Drawing for the job (mm, zero at the part's lowest x, y, z). A direction names the side the tool comes from. Give positions to 0.01 mm unless a question says otherwise; leave off trailing zeros. Loops run counter-clockwise (first coordinate to the right, second up) from the corner with the lowest first, then second, coordinate; pieces in that order, holes last. Notation, with made-up numbers: (52, -3) - (74, -3) arc R14 ccw to (74, 1) - close; hole circle Ø8 at (13, -28.75). An arc over 180 degrees is marked (long way). Return JSON: item names as keys, results as strings. Group by question number.
1) 3-axis set-ups, long thin cutter, end or side, ignore diameter. For the marked faces 4 and 5: which of +Z, -Z, +X, -X, +Y, -Y reach the whole face in a straight line?
2) Slice it at A-A (z = 41.5). List the corners of the cut face in (x, y).
3) Slice it at C-C (y = 70). List the corners of the cut face in (x, z).
4) Slice it at B-B (x = 12.75). List the corners of the cut face in (y, z).
5) Drop flat-ended pins along their axis: pin 1 (8 mm diameter, centred on y = 73.5, z = 39.5, fed in from +X); pin 2 (5 mm diameter, centred on x = 3, z = 40.5, fed in from -Y). Give the stop position or say it passes through.
6) Mould opens along Y. For the marked faces 1, 2 and 3 say: released by +Y, released by -Y, zero draft, split by the parting line, or undercut.
7) Drill centre lines: probe 1 along Z at (x, y) = (11, 53.5); probe 2 along Y at (x, z) = (5, 90); probe 3 along X at (y, z) = (74, 47). Where is each one in solid material? Low to high. Write a range as from..to.
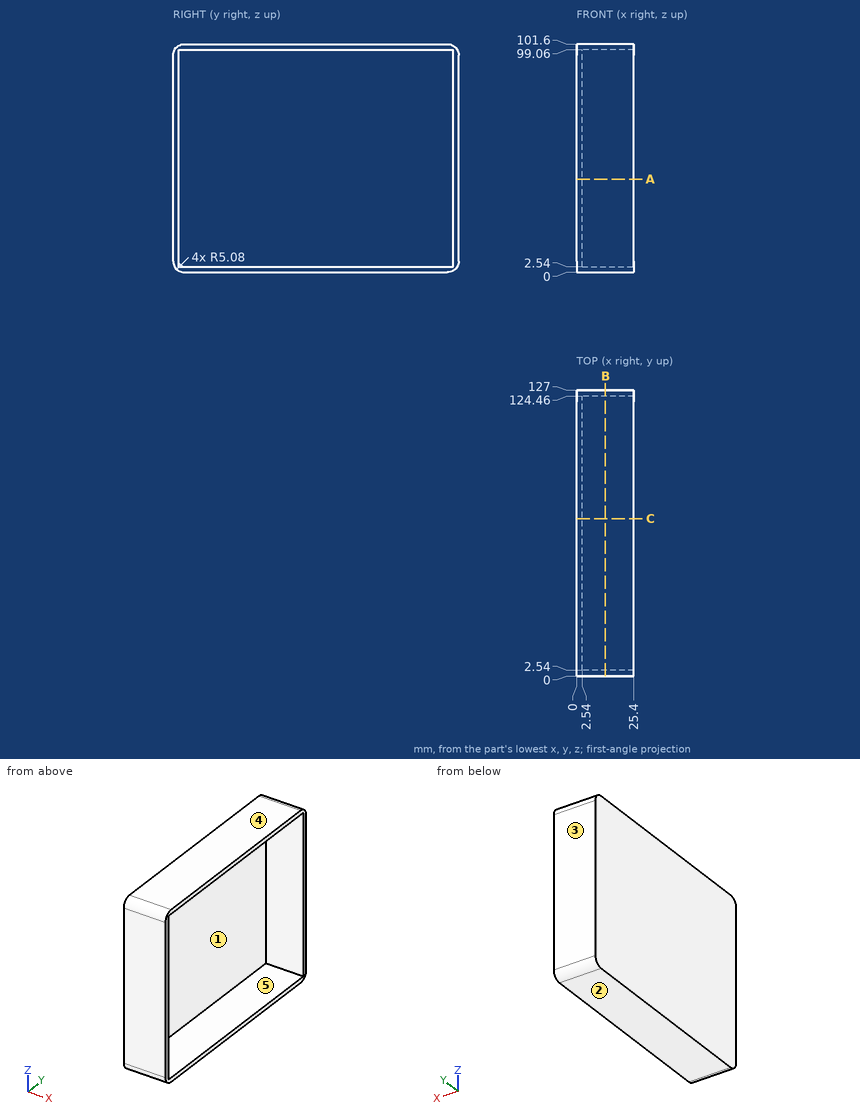
Results:
{
 "1": {"face 4": "+Z, +X, -X, +Y, -Y", "face 5": "+X"},
 "2": {"outline": "(0, 0) - (25.4, 0) - (25.4, 2.54) - (2.54, 2.54) - (2.54, 124.46) - (25.4, 124.46) - (25.4, 127) - (0, 127) - close"},
 "3": {"outline": "(0, 0) - (25.4, 0) - (25.4, 2.54) - (2.54, 2.54) - (2.54, 99.06) - (25.4, 99.06) - (25.4, 101.6) - (0, 101.6) - close"},
 "4": {"outline": "(0, 5.08) arc R5.08 ccw to (5.08, 0) - (121.92, 0) arc R5.08 ccw to (127, 5.08) - (127, 96.52) arc R5.08 ccw to (121.92, 101.6) - (5.08, 101.6) arc R5.08 ccw to (0, 96.52) - close; hole (2.54, 2.54) - (124.46, 2.54) - (124.46, 99.06) - (2.54, 99.06) - close"},
 "5": {"pin 1": "x = 2.54", "pin 2": "y = 0"},
 "6": {"face 1": "undercut", "face 2": "zero draft", "face 3": "released by +Y"},
 "7": {"probe 1": "0..2.54, 99.06..101.6", "probe 2": "0..2.54, 124.46..127", "probe 3": "0..2.54"}
}
